```python
from build123d import *

# Parameters (mm, degrees)
BOSS_EXTRUDE1_START = 6.3
SKETCH1_R           = 1.95
BOSS_EXTRUDE1_DEPTH = 4
CHAMFER1_SIZE       = 13
CHAMFER2_SIZE       = 13
FILLET1_R           = 5
SKETCH2_R           = 1.525
CUT_EXTRUDE1_DEPTH  = 62.410503988


with BuildPart() as part:
    # Sketch1 → Boss-Extrude1 (new body)
    with BuildSketch(Plane(origin=(0, 0, 0), x_dir=(1, 0, 0), z_dir=(0, 1, 0)).offset(BOSS_EXTRUDE1_START)):
        with BuildLine():
            Line((-54.1, -5), (-54.1, -16.2))
            Line((-54.1, -16.2), (43.9, -16.2))
            Line((43.9, -16.2), (43.9, -5))
            ThreePointArc((43.9, -5), (48.9, 0), (43.9, 5))
            Line((43.9, 5), (24.9, 5))
            Line((24.9, 5), (24.9, -6.2))
            Line((24.9, -6.2), (-35.1, -6.2))
            Line((-35.1, -6.2), (-35.1, 5))
            Line((-35.1, 5), (-54.1, 5))
            ThreePointArc((-54.1, 5), (-59.1, 0), (-54.1, -5))
        make_face()
        with Locations(Location((43.9, 0, 0), (0, 0, 90))):
            Circle(SKETCH1_R, mode=Mode.SUBTRACT)
        with Locations(Location((-54.1, 0, 0), (0, 0, 90))):
            Circle(SKETCH1_R, mode=Mode.SUBTRACT)
    extrude(amount=BOSS_EXTRUDE1_DEPTH)

    # Chamfer1
    # the kernel refuses this chamfer: 13 mm, written as the material it takes off along each edge
    with BuildSketch(Plane(origin=(24.9, -27.131878844, -5), x_dir=(0.9996219169112968, 0, -0.027495876610586358), z_dir=(0, 1, 0))) as chamfer1_piece_1_section:
        Polygon((CHAMFER1_SIZE * 0.999621916911, -CHAMFER1_SIZE * 0.0274958766106), (-CHAMFER1_SIZE * 0.0274958766106, -CHAMFER1_SIZE * 0.999621916911), (0, 0), align=None)
    chamfer1_piece_1 = extrude(amount=70.863757687, mode=Mode.PRIVATE)
    chamfer1_piece_1 = split(chamfer1_piece_1, bisect_by=Plane(origin=(29.309865353, 8.3, 6.2), z_dir=(0, 0, -1)), keep=Keep.TOP, mode=Mode.PRIVATE)
    add(chamfer1_piece_1, mode=Mode.SUBTRACT)
    with BuildSketch(Plane(origin=(-35.1, -27.131878844, -5), x_dir=(0.027495876610586424, 0, 0.9996219169112968), z_dir=(0, 1, 0))) as chamfer1_piece_2_section:
        Polygon((CHAMFER1_SIZE * 0.999621916911, -CHAMFER1_SIZE * 0.0274958766106), (-CHAMFER1_SIZE * 0.0274958766106, -CHAMFER1_SIZE * 0.999621916911), (0, 0), align=None)
    chamfer1_piece_2 = extrude(amount=70.863757687, mode=Mode.PRIVATE)
    chamfer1_piece_2 = split(chamfer1_piece_2, bisect_by=Plane(origin=(-39.509865353, 8.3, 6.2), z_dir=(0, 0, -1)), keep=Keep.TOP, mode=Mode.PRIVATE)
    add(chamfer1_piece_2, mode=Mode.SUBTRACT)

    # Chamfer2
    # the kernel refuses this chamfer: 13 mm, written as the material it takes off along each edge
    with BuildSketch(Plane(origin=(43.9, -27.131878844, 16.2), x_dir=(0.02749587661058749, 0, -0.9996219169112966), z_dir=(0, 1, 0))) as chamfer2_piece_1_section:
        Polygon((CHAMFER2_SIZE * 0.999621916911, CHAMFER2_SIZE * 0.0274958766106), (-CHAMFER2_SIZE * 0.0274958766106, CHAMFER2_SIZE * 0.999621916911), (0, 0), align=None)
    chamfer2_piece_1 = extrude(amount=70.863757687, mode=Mode.PRIVATE)
    chamfer2_piece_1 = chamfer2_piece_1 - Plane(origin=(43.9, 8.3, 0), x_dir=(0, 0, 1), z_dir=(0, -1, 0)) * Cylinder(5, 194, mode=Mode.PRIVATE)
    add(chamfer2_piece_1, mode=Mode.SUBTRACT)
    with BuildSketch(Plane(origin=(-54.1, -27.131878844, 16.2), x_dir=(-0.027495876610587482, 0, -0.9996219169112966), z_dir=(0, 1, 0))) as chamfer2_piece_2_section:
        Polygon((CHAMFER2_SIZE * 0.999621916911, -CHAMFER2_SIZE * 0.0274958766106), (-CHAMFER2_SIZE * 0.0274958766106, -CHAMFER2_SIZE * 0.999621916911), (0, 0), align=None)
    chamfer2_piece_2 = extrude(amount=70.863757687, mode=Mode.PRIVATE)
    chamfer2_piece_2 = chamfer2_piece_2 - Plane(origin=(-54.1, 8.3, 0), x_dir=(0, 0, -1), z_dir=(0, -1, 0)) * Cylinder(5, 194, mode=Mode.PRIVATE)
    add(chamfer2_piece_2, mode=Mode.SUBTRACT)

    # Fillet1
    fillet1_edges = [part.edges().sort_by_distance(p)[0] for p in [
        (42.347223446, 8.3, 4.752776554),
        (-52.547223446, 8.3, 4.752776554),
        (37.9, 8.3, -5),
        (-48.1, 8.3, -5),
        (26.7, 8.3, 6.2),
        (-36.9, 8.3, 6.2),
        (-41.1, 8.3, 16.2),
        (30.9, 8.3, 16.2),
    ]]
    fillet(fillet1_edges, radius=FILLET1_R)

    # Sketch2 → Cut-Extrude1 (cut, through all)
    with BuildSketch(Plane(origin=(0, 10.3, 0), x_dir=(1, 0, 0), z_dir=(0, 1, 0))):
        with Locations(Location((29.9, -10.1, 0), (0, 0, 270))):
            Circle(SKETCH2_R)
        with Locations(Location((-5.1, -11.2, 0), (0, 0, 270))):
            Circle(SKETCH2_R)
        with Locations(Location((9.9, -11.2, 0), (0, 0, 270))):
            Circle(SKETCH2_R)
        with Locations(Location((-40.1, -10.1, 0), (0, 0, 90))):
            Circle(SKETCH2_R)
        with Locations(Location((-20.1, -11.2, 0), (0, 0, 90))):
            Circle(SKETCH2_R)
        with Locations(Location((19.9, -11.2, 0), (0, 0, 270))):
            Circle(SKETCH2_R)
        with Locations(Location((-30.1, -11.2, 0), (0, 0, 90))):
            Circle(SKETCH2_R)
    extrude(amount=-CUT_EXTRUDE1_DEPTH, mode=Mode.SUBTRACT)


solid = part.part
```
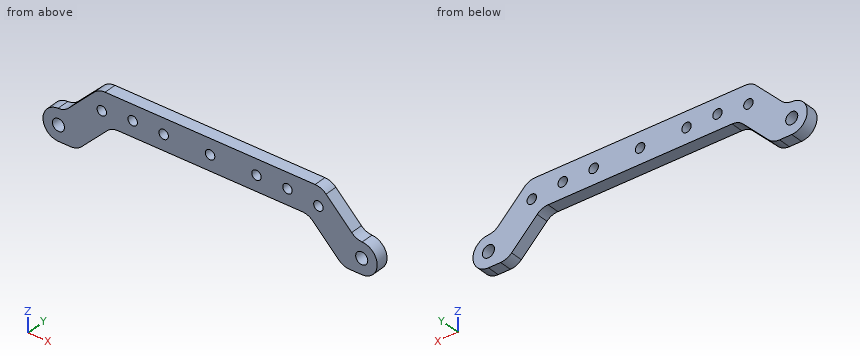
Design review of the part built by this model. Coordinates are the model's own, in mm. Coordinates: 2 decimals unless noted, no trailing zeros. Order: outer loops, then holes, each group sorted by start corner. A loop starts at its lowest first (then second) coordinate and runs counter-clockwise, first axis right, second up. Notation, with made-up numbers: (83, 46) - (122, 46) arc R18 ccw to (122, 62) - close; hole circle Ø3 at (-17, 7.5). An arc over 180 degrees is marked (long way). Answer in a Markdown table with one row per item.
(1) Wall thickness on line 1 along Z through (x, y) = (-54.1, 7.7); line 2 along Z through (x, y) = (-20.1, 7.9) (3 decimals); line 3 along X through (y, z) = (8.05, 0.5): over which ranges is each line inside the solid? List them lowest first. Write a range as from..to.
Checked values:
| item | result |
|---|---|
| line 1 | -5..-1.95, 1.95..5 |
| line 2 | 6.2..9.675, 12.725..16.2 |
| line 3 | -59.07..-55.98, -52.22..-42.6, 32.4..42.02, 45.78..48.87 |
(2) Consider section D-D on x = 3.5. State the section outline as (y, z) points, plus the area to 3 significant figures.
Checked values:
| item | result |
|---|---|
| outline | (6.3, 6.2) - (10.3, 6.2) - (10.3, 16.2) - (6.3, 16.2) - close |
| area | 40.0 mm^2 |
(3) Consider section C-C on y = 9.1. Give the number of separate pieces and of enclosed holes in the cut face, plus the area to 3 significant figures.
Checked values:
| item | result |
|---|---|
| separate pieces | 1 |
| enclosed holes | 9 |
| area | 1,080 mm^2 |
(4) Consider section B-B on z = 0. State the section outline as (x, y) points.
Checked values:
| item | result |
|---|---|
| outline | (-59.1, 6.3) - (-56.05, 6.3) - (-56.05, 10.3) - (-59.1, 10.3) - close; (-52.15, 6.3) - (-43.1, 6.3) - (-43.1, 10.3) - (-52.15, 10.3) - close; (32.9, 6.3) - (41.95, 6.3) - (41.95, 10.3) - (32.9, 10.3) - close; (45.85, 6.3) - (48.9, 6.3) - (48.9, 10.3) - (45.85, 10.3) - close |
(5) Consider section A-A on x = 19.9. State the section outline as (y, z) points (3 decimals), plus the area to 3 significant figures.
Checked values:
| item | result |
|---|---|
| outline | (6.3, 6.2) - (10.3, 6.2) - (10.3, 9.675) - (6.3, 9.675) - close; (6.3, 12.725) - (10.3, 12.725) - (10.3, 16.2) - (6.3, 16.2) - close |
| area | 27.8 mm^2 |
